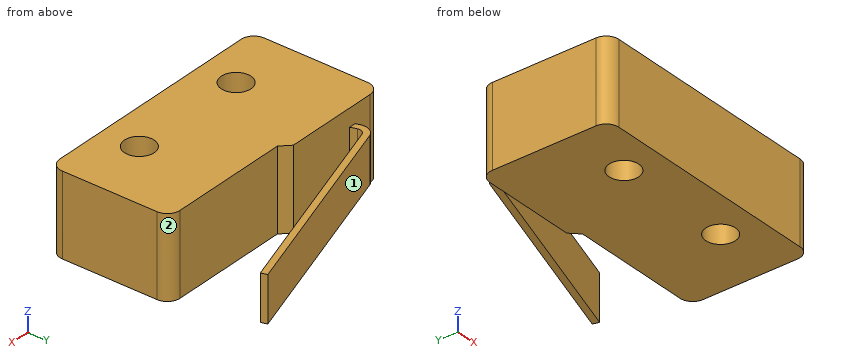
```python
from build123d import *

# Parameters (mm, degrees)
ESQUISSE1_R        = 1.175
BOSS_EXTRU_1_DEPTH = 6.4
BOSS_EXTRU_2_DEPTH = 3.6


with BuildPart() as part:
    # Esquisse1 → Boss.-Extru.1 (new body)
    with BuildSketch(Plane.XY):
        with BuildLine():
            Line((1, 0), (18.8, 0))
            ThreePointArc((18.8, 0), (19.507106781, 0.292893219), (19.8, 1))
            Line((19.8, 1), (19.8, 8.5))
            ThreePointArc((19.8, 8.5), (19.507106781, 9.207106781), (18.8, 9.5))
            Line((18.8, 9.5), (9.235956187, 9.5))
            Line((9.235956187, 9.5), (8.535956187, 10.2))
            Line((8.535956187, 10.2), (1, 10.2))
            ThreePointArc((1, 10.2), (0.292893219, 9.907106781), (0, 9.2))
            Line((0, 9.2), (0, 1))
            ThreePointArc((0, 1), (0.292893219, 0.292893219), (1, 0))
        make_face()
        with Locations((5.1, 2.9)):
            Circle(ESQUISSE1_R, mode=Mode.SUBTRACT)
        with Locations((14.6, 2.9)):
            Circle(ESQUISSE1_R, mode=Mode.SUBTRACT)
    extrude(amount=BOSS_EXTRU_1_DEPTH)

    # Esquisse2 → Boss.-Extru.2 (add)
    with BuildSketch(Plane.XY.offset(5)):
        with BuildLine():
            Line((2.475579427, 10.2), (2.372481297, 10.525914526))
            ThreePointArc((2.372481297, 10.525914526), (2.438469066, 11.288431445), (3.024310349, 11.780951931))
            Line((3.024310349, 11.780951931), (19.449197912, 16.976716614))
            Line((19.449197912, 16.976716614), (19.6, 16.5))
            Line((19.6, 16.5), (3.175112437, 11.304235317))
            ThreePointArc((3.175112437, 11.304235317), (2.882191796, 11.057975074), (2.849197912, 10.676716614))
            Line((2.849197912, 10.676716614), (3, 10.2))
            Line((3, 10.2), (2.475579427, 10.2))
        make_face()
    extrude(amount=-BOSS_EXTRU_2_DEPTH)


solid = part.part
```
Geometry: final body of the model. Coordinates: model frame, mm. Face numbers are marked on the shaded views. A direction names the side the tool comes from. Coordinates: 2 decimals unless noted, no trailing zeros. Order: outer loops, then holes, each group sorted by start corner. A loop starts at its lowest first (then second) coordinate and runs counter-clockwise, first axis right, second up. Notation, with made-up numbers: M 33.25,35 L 50.25,35 A18 ccw 50.25,65 Z; hole C 60.25,11.25 d4. An arc over 180 degrees is marked long. Answer as CSV lines item,"result".
Q1. Section B-B on x = 7. Return the cut outline in (y, z), and give its area (3 significant figures).
Answers:
outline,"M 0,0 L 10.2,0 L 10.2,6.4 L 0,6.4 Z; M 12.51,1.4 L 13.04,1.4 L 13.04,5 L 12.51,5 Z"
area,"67.2 mm^2"
Q2. Set-up query: the marked faces 1 and 2. Return all of +Z, -Z, +X, -X, +Y, -Y with unobstructed straight access to the full face (end or side cutting, diameter ignored); none if empty.
Answers:
face 1,"+Z, -Z, -X, +Y"
face 2,"+Z, -Z, +X"
Q3. Section C-C on z = 5.5. Return the cut outline in (x, y) (3 decimals), and give its area (3 significant figures).
Answers:
outline,"M 0,1 A1 ccw 1,0 L 18.8,0 A1 ccw 19.8,1 L 19.8,8.5 A1 ccw 18.8,9.5 L 9.236,9.5 L 8.536,10.2 L 1,10.2 A1 ccw 0,9.2 Z; hole C 5.1,2.9 d2.35; hole C 14.6,2.9 d2.35"
area,"185 mm^2"
Q4. First-contact query: P1, Ø3.5, axis at x = 14.5, y = 14.5, coming from the +Z side; P2, Ø1.9, axis at x = 5, z = 2, coming from the +Y side; P3, Ø3, axis at x = 2.5, z = 5, coming from the +Y side. Flat tips, straight axial feed; report the tip coordinate or a pass-through.
Answers:
P1,"stops at z = 5"
P2,"stops at y = 12.71"
P3,"stops at y = 12.09"
Q5. Section D-D on x = 14.6. Return the cut outline in (y, z) (3 decimals).
Answers:
outline,"M 0,0 L 1.725,0 L 1.725,6.4 L 0,6.4 Z; M 4.075,0 L 9.5,0 L 9.5,6.4 L 4.075,6.4 Z; M 14.918,1.4 L 15.443,1.4 L 15.443,5 L 14.918,5 Z"
Q6. Line query: probe 1 along Y at (x, z) = (14.5, 3.5); probe 2 along X at (y, z) = (3.25, 2); probe 3 along X at (y, z) = (3.5, 1.5). Output: solid intervals per line, ascending. Write a range as [from, to].
Answers:
probe 1,"y = [0, 1.73], [4.07, 9.5], [14.89, 15.41]"
probe 2,"x = [0, 3.98], [6.22, 13.48], [15.72, 19.8]"
probe 3,"x = [0, 4.09], [6.11, 13.59], [15.61, 19.8]"
Q7. Section A-A on y = 2.9. Return the cut outline in (x, z) (3 decimals), and give its area (3 significant figures).
Answers:
outline,"M 0,0 L 3.925,0 L 3.925,6.4 L 0,6.4 Z; M 6.275,0 L 13.425,0 L 13.425,6.4 L 6.275,6.4 Z; M 15.775,0 L 19.8,0 L 19.8,6.4 L 15.775,6.4 Z"
area,"96.6 mm^2"
